```python
from build123d import *

# Parameters (mm, degrees)
BASE_FLANGE1_DEPTH = 254
SKETCH7_R          = 3.175
CUT_EXTRUDE1_DEPTH = 274.495613128


# Sheet-metal steps are written as plain solids
with BuildPart() as part:
    # Sketch2 → Base-Flange1 (new body)
    with BuildSketch(Plane.XY):
        with BuildLine():
            Line((0, 38.1), (0, 3.175))
            ThreePointArc((0, 3.175), (0.92993597, 0.92993597), (3.175, 0))
            Line((3.175, 0), (85.725, 0))
            ThreePointArc((85.725, 0), (87.97006403, 0.92993597), (88.9, 3.175))
            Line((88.9, 3.175), (88.9, 38.1))
            Line((88.9, 38.1), (91.44, 38.1))
            Line((91.44, 38.1), (91.44, 3.175))
            ThreePointArc((91.44, 3.175), (89.766115254, -0.866115254), (85.725, -2.54))
            Line((85.725, -2.54), (3.175, -2.54))
            ThreePointArc((3.175, -2.54), (-0.866115254, -0.866115254), (-2.54, 3.175))
            Line((-2.54, 3.175), (-2.54, 38.1))
            Line((-2.54, 38.1), (0, 38.1))
        make_face()
    extrude(amount=BASE_FLANGE1_DEPTH)

    # Sketch7 → Cut-Extrude1 (cut, through all)
    with BuildSketch(Plane(origin=(91.44, 0, 0), x_dir=(0, 0, -1), z_dir=(1, 0, 0))):
        with Locations(Location((-165.1, 25.4, 0), (0, 0, 90))):
            Circle(SKETCH7_R)
        Polygon((-254, 38.1), (-254, 3.175), (-177.8, 38.1), align=None)
        Polygon((0, 38.1), (0, 3.175), (-152.4, 38.1), align=None)
    extrude(amount=-CUT_EXTRUDE1_DEPTH, mode=Mode.SUBTRACT)


solid = part.part
```
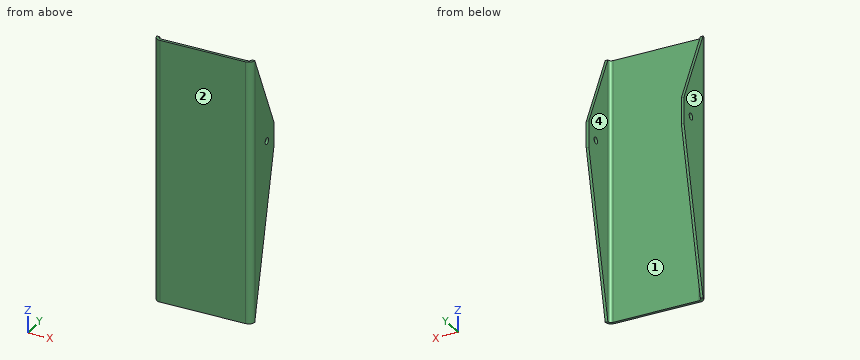
Can you work these out from the model? Positions are in its coordinate system, mm. Face numbers are marked on the shaded views. Round coordinates to 2 decimals unless told otherwise and drop trailing zeros. Order: outer loops, then holes, each group sorted by start corner. A loop starts at its lowest first (then second) coordinate and runs counter-clockwise, first axis right, second up.
(1) If we section it at A-A (z = 165.1): Please give me the cut outline in (x, y) (3 decimals).
Results are:
outline: (-2.54, 3.175) arc R5.715 ccw to (3.175, -2.54) - (85.725, -2.54) arc R5.715 ccw to (91.44, 3.175) - (91.44, 22.225) - (88.9, 22.225) - (88.9, 3.175) arc R3.175 cw to (85.725, 0) - (3.175, 0) arc R3.175 cw to (0, 3.175) - (0, 22.225) - (-2.54, 22.225) - close; (-2.54, 28.575) - (0, 28.575) - (0, 38.1) - (-2.54, 38.1) - close; (88.9, 28.575) - (91.44, 28.575) - (91.44, 38.1) - (88.9, 38.1) - close
(2) We'd pull the mould along X, two halves only. Please class the marked faces 1, 2, 3 and 4: +X half, -X half, draft (parallel to the pull), parting line (faces both ways), or undercut.
Results are:
face 1: undercut
face 2: draft
face 3: -X half
face 4: undercut
(3) I'm going to push flat-ended pins straight in: pin 1 (1.5 mm diameter, centred on x = 27, z = 137.5, fed in from +Y); pin 2 (4 mm diameter, centred on y = 25.4, z = 165.1, fed in from -X). Where does each tip first touch, or does it pass through?
Results are:
pin 1: stops at y = 0
pin 2: passes through
(4) If we section it at C-C (y = 11): Please give me the cut outline in (x, z), plus the area to 3 significant figures.
Results are:
outline: (-2.54, 34.15) - (0, 34.15) - (0, 236.93) - (-2.54, 236.93) - close; (88.9, 34.15) - (91.44, 34.15) - (91.44, 236.93) - (88.9, 236.93) - close
area: 1,030 mm2
(5) If I drill on L1, parallel to X at y = 15.5, z = 225.5; L2, parallel to Y at x = 70, z = 135.5; L3, parallel to Y at x = -1.85, z = 165.1 (3 decimals), over which ranges is the centre line in solid material (lowest first)?
Results are:
L1: x = -2.54 to 0, 88.9 to 91.44
L2: y = -2.54 to 0
L3: y = 0.453 to 22.225, 28.575 to 38.1
(6) If we section it at D-D (x = 58.5): Please give me the cut outline in (y, z).
Results are:
outline: (-2.54, 0) - (0, 0) - (0, 254) - (-2.54, 254) - close
(7) If we section it at B-B (y = 25.4): Please give me the cut outline in (x, z) (3 decimals), plus the area to 3 significant figures.
Results are:
outline: (-2.54, 96.982) - (0, 96.982) - (0, 161.925) - (-2.54, 161.925) - close; (-2.54, 168.275) - (0, 168.275) - (0, 205.509) - (-2.54, 205.509) - close; (88.9, 96.982) - (91.44, 96.982) - (91.44, 161.925) - (88.9, 161.925) - close; (88.9, 168.275) - (91.44, 168.275) - (91.44, 205.509) - (88.9, 205.509) - close
area: 519 mm2
